from build123d import *

# Parameters (mm, degrees)
F0_W          = 200
F0_H          = 4
F1_DEPTH      = 1.4
F2_R          = 1.99999
F5_DEPTH      = 1.775
F6_SIZE       = 0.75
F7_DEPTH      = 1.4
F7_DEPTH_BACK = 25


# Not quite as in the source:
# - a fillet or chamfer is up to 0.001 mm smaller than in the source, because OpenCascade refuses the exact size


with BuildPart() as f1:
    # F0 (on Top) → F1 (new body)
    with BuildSketch(Plane.XY):
        with Locations((100, 2)):
            Rectangle(F0_W, F0_H)
    extrude(amount=F1_DEPTH)

    # F2 (radius 2 in the source; OpenCascade refuses exactly that, so slightly less here)
    f2_edges = [f1.edges().sort_by_distance(p)[0] for p in [
        (0, 0, 0.7),
        (0, 4, 0.7),
        (200, 0, 0.7),
        (200, 4, 0.7),
    ]]
    fillet(f2_edges, radius=F2_R)

    # F4 (on face) → F5 (join)
    with BuildSketch(Plane.XY.offset(1.4)):
        with BuildLine():
            Line((198, 5), (2, 5))
            ThreePointArc((2, 5), (-1, 2), (2, -1))
            Line((2, -1), (198, -1))
            ThreePointArc((198, -1), (201, 2), (198, 5))
        make_face()
    extrude(amount=F5_DEPTH)

    # F6
    f6_edges = [f1.edges().sort_by_distance(p)[0] for p in [
        (-1, 2, 3.175),
    ]]
    chamfer(f6_edges, length=F6_SIZE)

    # F3 (on face) → F7 (cut, two sides)
    with BuildSketch(Plane.XY.offset(1.4)) as f7_sk:
        Polygon((18, 3.5875), (18, 2), (18, 0.4125), (33.875, 0.4125), (33.875, 3.5875), align=None)
        Polygon((182, 0.4125), (182, 2), (182, 3.5875), (166.125, 3.5875), (166.125, 0.4125), align=None)
        Polygon((92.0625, 3.5875), (92.0625, 2), (92.0625, 0.4125), (107.9375, 0.4125), (107.9375, 3.5875), align=None)
    extrude(amount=-F7_DEPTH, mode=Mode.SUBTRACT)
    extrude(f7_sk.sketch, amount=F7_DEPTH_BACK, mode=Mode.SUBTRACT)


solid = f1.part
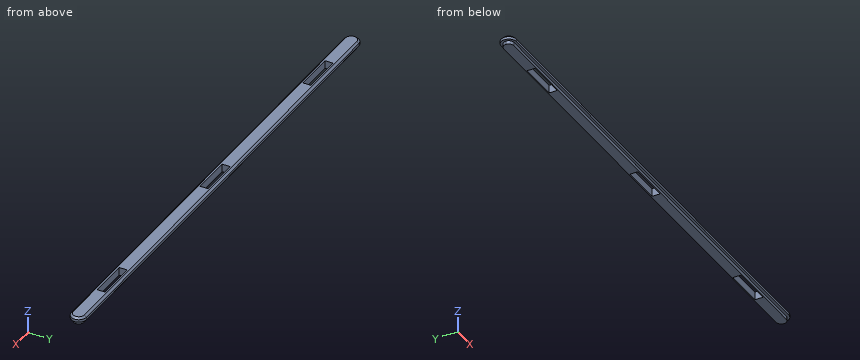
Geometry check sheet. Reference: the model listing, model coordinates, mm. Round coordinates to 2 decimals unless told otherwise and drop trailing zeros. Loops run counter-clockwise (first coordinate to the right, second up) from the corner with the lowest first, then second, coordinate; pieces in that order, holes last. Notation, with made-up numbers: (39, -12.75) -> (92, -12.75) arc R5 cw to (92, -3.75) -> close; hole circle Ø1 at (53.5, 19). An arc over 180 degrees is marked (long way). Answer as a JSON object with one key per item and string values. Group by question number.
Item 1: Thickness scan on line 1 along X through (y, z) = (2.45, 2.4) (1 decimal); line 2 along X through (y, z) = (2.3, 0.3) (1 decimal); line 3 along Y through (x, z) = (21, 0.2). Record the ranges inside material, lowest first.
Item 2: Cross-section at A-A, the plane z = 1.9. Record the cut outline in (x, y) (1 decimal).
Item 3: Depth check by flat-ended pin: pin 1 Ø1.1 at (x, z) = (124.5, 0.5) entering from -Y; pin 2 Ø1.5 at (x, z) = (118.5, 0.5) entering from +Y. Enter the tip coordinate at first touch or a pass-through.
Item 4: Cross-section at B-B, the plane x = 38. Record the cut outline in (y, z) (3 decimals).
Determined:
{
 "1": {"line 1": "x = -1 to 18, 33.9 to 92.1, 107.9 to 166.1, 182 to 201", "line 2": "x = 0 to 18, 33.9 to 92.1, 107.9 to 166.1, 182 to 200", "line 3": "y = 0 to 0.41, 3.59 to 4"},
 "2": {"outline": "(2, -1) -> (198, -1) arc R3 ccw to (198, 5) -> (2, 5) arc R3 ccw to start; hole (18, 0.4) -> (33.9, 0.4) -> (33.9, 3.6) -> (18, 3.6) -> close; hole (92.1, 0.4) -> (107.9, 0.4) -> (107.9, 3.6) -> (92.1, 3.6) -> close; hole (166.1, 0.4) -> (182, 0.4) -> (182, 3.6) -> (166.1, 3.6) -> close"},
 "3": {"pin 1": "stops at y = 0", "pin 2": "stops at y = 4"},
 "4": {"outline": "(-1, 1.4) -> (0, 1.4) -> (0, 0) -> (4, 0) -> (4, 1.4) -> (5, 1.4) -> (5, 2.425) -> (4.25, 3.175) -> (-0.25, 3.175) -> (-1, 2.425) -> close"}
}
